Check sheet for the drawn part. Datum: minimum x, y, z corner. Units: mm. A direction names the side the tool comes from. Coordinates: 2 decimals unless noted, no trailing zeros. Loops run counter-clockwise (first coordinate to the right, second up) from the corner with the lowest first, then second, coordinate; pieces in that order, holes last.
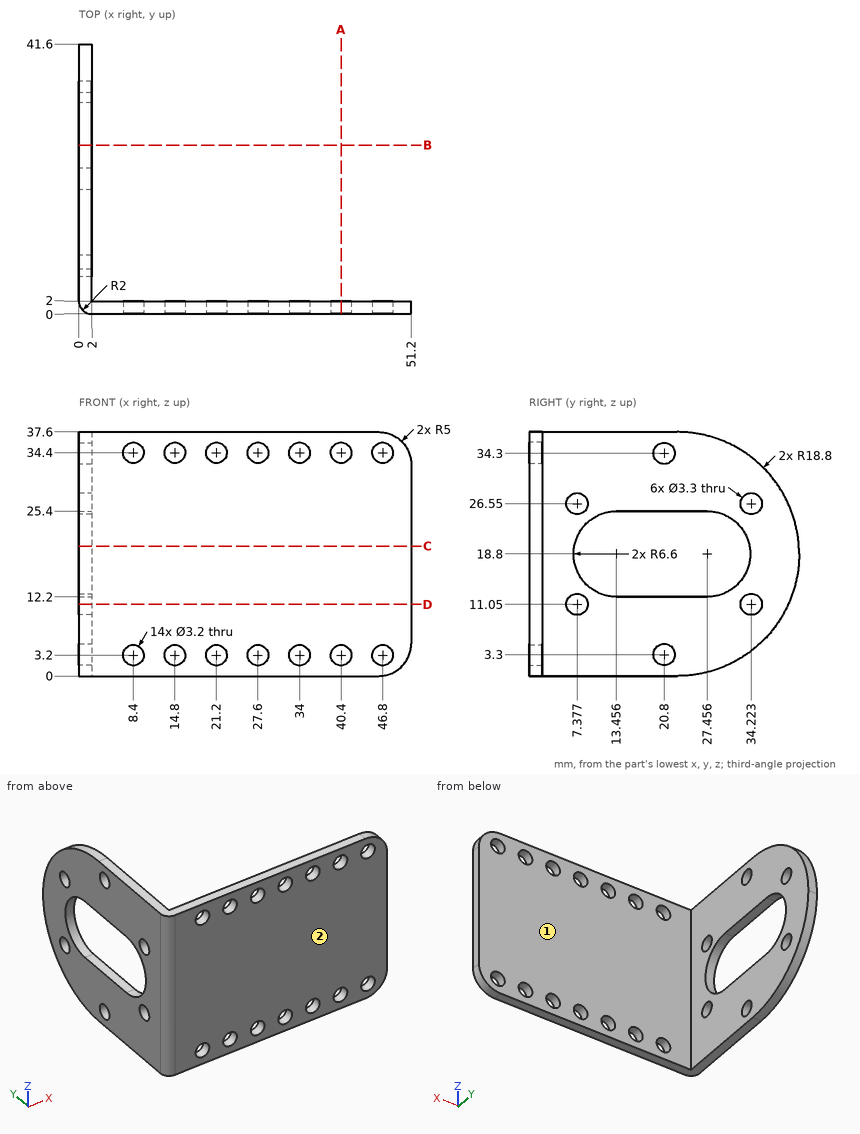
(1) Gauge pin test, flat ends, axial feed: pin 1 Ø3.5 at (x, z) = (34, 3.2) entering from +Y; pin 2 Ø11.5 at (y, z) = (26.5, 10) entering from +X. Record the tip position at first contact, or that the pin passes through.
Findings:
pin 1: stops at y = 2
pin 2: stops at x = 2
(2) Sectioned sample at D-D on z = 11.05. Record the cut outline in (x, y).
Findings:
outline: (0, 2) arc R2 ccw to (2, 0) - (51.2, 0) - (51.2, 2) - (2, 2) - (2, 5.73) - (0, 5.73) - close; (0, 9.03) - (2, 9.03) - (2, 32.57) - (0, 32.57) - close; (0, 35.87) - (2, 35.87) - (2, 39.93) - (0, 39.93) - close
(3) Access from +Z, -Z, +X, -X, +Y, -Y to the whole of each face (thin tool, end or side, straight path). Record for the marked faces 1 and 2.
Findings:
face 1: +Z, -Z, +X, +Y
face 2: +Z, -Z, +X, -X, -Y
(4) Scan lines: L1, parallel to X at y = 30, z = 34.5; L2, parallel to Z at x = 40, y = 1. Record each from-to range of solid material in increasing order.
Findings:
L1: x = 0 to 2
L2: z = 0 to 1.65, 4.75 to 32.85, 35.95 to 37.6
(5) Sectioned sample at A-A on x = 40.4. Record the cut outline in (y, z).
Findings:
outline: (0, 0) - (2, 0) - (2, 1.6) - (0, 1.6) - close; (0, 4.8) - (2, 4.8) - (2, 32.8) - (0, 32.8) - close; (0, 36) - (2, 36) - (2, 37.6) - (0, 37.6) - close
(6) Sectioned sample at C-C on z = 20. Record the cut outline in (x, y), and give its area (3 significant figures).
Findings:
outline: (0, 2) arc R2 ccw to (2, 0) - (51.2, 0) - (51.2, 2) - (2, 2) - (2, 6.97) - (0, 6.97) - close; (0, 33.95) - (2, 33.95) - (2, 41.56) - (0, 41.56) - close
area: 127 mm2
(7) Sectioned sample at B-B on y = 26. Record the cut outline in (x, z) (1 decimal).
Findings:
outline: (0, 0.3) - (2, 0.3) - (2, 12.2) - (0, 12.2) - close; (0, 25.4) - (2, 25.4) - (2, 37.3) - (0, 37.3) - close
